```python
from build123d import *

# Parameters (mm, degrees)
CUT_EXTRUDE1_DEPTH = 6.35
CHAMFER1_SIZE      = 0.762


with BuildPart() as part:
    # Sketch1 → Base-Revolve (revolve)
    with BuildSketch(Plane.XY, mode=Mode.PRIVATE) as base_revolve_sk:
        Polygon((4.7625, 0), (7.14375, 0), (7.14375, 9.525), (0, 9.525), (0, -31.75), (4.7625, -31.75), align=None)
    revolve(base_revolve_sk.sketch.rotate(Axis((0, 0, 0), (0, 1, 0)), 90), axis=Axis((0, 0, 0), (0, 1, 0)))

    # Sketch2 → Cut-Extrude1 (cut)
    with BuildSketch(Plane(origin=(0, 9.525, 0), x_dir=(-1, 0, 0), z_dir=(0, 1, 0))):
        Polygon((2.291358881, -3.96875), (-2.291358881, -3.96875), (-4.582717762, 0), (-2.291358881, 3.96875), (2.291358881, 3.96875), (4.582717762, 0), align=None)
    extrude(amount=-CUT_EXTRUDE1_DEPTH, mode=Mode.SUBTRACT)

    # Chamfer1
    chamfer1_edges = [part.edges().sort_by_distance(p)[0] for p in [
        (0, 9.525, 7.14375),
    ]]
    chamfer(chamfer1_edges, length=CHAMFER1_SIZE)


solid = part.part
```
Here's how the part is built. I have some questions about the finished solid (model axes, mm). A direction names the side the tool comes from. Give positions to 0.01 mm unless a question says otherwise; leave off trailing zeros. Write each loop counter-clockwise with the first axis right and the second up, starting at its lowest first coordinate (ties: lowest second). Pieces come first, ordered by that corner, then holes. Notation, with made-up numbers: (15, 28) -> (23, 28) arc R37 cw to (23, 66) -> close; hole circle Ø7 at (16, -10). An arc over 180 degrees is marked (long way). Write each question's results on one line, items separated by ' | '.
Item 1: We'd pull the mould along Z, two halves only. Please class faces 4 (the face through (3.42, 6.39, -2.01)), 5 (the face through (-0.314, 4.443, 7.137)), 6 (the face through (0, -31.75, 0)): pulls with the +Z half, pulls with the -Z half, needs draft (parallel to the pull), parting line crosses it, or undercut.
Output:
face 4: undercut | face 5: parting line crosses it | face 6: needs draft
Item 2: For pin 1 Ø3 at (y, z) = (-2, 2) entering from +X; pin 2 Ø2.5 at (x, z) = (1, -0.5) entering from +Y (3 decimals); pin 3 Ø3 at (y, z) = (-13, -4.5) entering from +X, each with a flat end and sliding along its axis, tell me the tip position at first contact or that it passes through.
Output:
pin 1: stops at x = 4.74 | pin 2: stops at y = 3.175 | pin 3: stops at x = 3.7
Item 3: On a 3-axis mill with a long thin cutter (end or side, diameter ignored), from which of +Z, -Z, +X, -X, +Y, -Y can I reach the whole of each face in a straight line? I mean faces 1 (the face through (3.45, 6.39, 1.96)), 2 (the face through (-0.1, 9.525, -4.2)), 3 (the face through (1, 0, 5)). Say none if no direction works.
Output:
face 1: +Y | face 2: +Z, -Z, +X, -X, +Y | face 3: -Y
Item 4: If I drill on L1, parallel to Y at x = -5, z = 3 (3 decimals); L2, parallel to Y at x = -3.75, z = 0.25 (3 decimals); L3, parallel to Z at x = 2.5, y = 4.5, over which ranges is the centre line in solid material (lowest first)?
Output:
L1: y = 0 to 9.525 | L2: y = -31.75 to 3.175 | L3: z = -6.69 to -3.61, 3.61 to 6.69
Item 5: Suppose I cut it at B-B on y = -2. Write out the boundary of the cut face in (x, z) (1 decimal), plus the area to 3 significant figures.
Output:
outline: circle Ø9.5 at (0, 0) | area: 71.3 mm^2
